from build123d import *

# Parameters (mm, degrees)
SKETCH1_R           = 2.5
BOSS_EXTRUDE1_DEPTH = 10


with BuildPart() as part:
    # Sketch1 → Boss-Extrude1 (new body)
    with BuildSketch(Plane.XY):
        with BuildLine():
            Line((-30, 0), (-22.5, 0))
            Line((-22.5, 0), (-22.5, 1))
            ThreePointArc((-22.5, 1), (-22.207106781, 1.707106781), (-21.5, 2))
            Line((-21.5, 2), (-9, 2))
            Line((-9, 2), (-9, 3))
            ThreePointArc((-9, 3), (-8.707106781, 3.707106781), (-8, 4))
            Line((-8, 4), (8, 4))
            ThreePointArc((8, 4), (8.707106781, 3.707106781), (9, 3))
            Line((9, 3), (9, 2))
            Line((9, 2), (21.5, 2))
            ThreePointArc((21.5, 2), (22.207106781, 1.707106781), (22.5, 1))
            Line((22.5, 1), (22.5, 0))
            Line((22.5, 0), (30, 0))
            Line((30, 0), (24.933748499, 30.8112495))
            ThreePointArc((24.933748499, 30.8112495), (23.236027851, 33.811577593), (20, 35))
            Line((20, 35), (16, 35))
            Line((16, 35), (16, 29))
            ThreePointArc((16, 29), (15.414213562, 27.585786438), (14, 27))
            Line((14, 27), (10, 27))
            ThreePointArc((10, 27), (0, 17), (-10, 27))
            Line((-10, 27), (-14, 27))
            ThreePointArc((-14, 27), (-15.414213562, 27.585786438), (-16, 29))
            Line((-16, 29), (-16, 35))
            Line((-16, 35), (-20, 35))
            ThreePointArc((-20, 35), (-23.236027851, 33.811577593), (-24.933748499, 30.8112495))
            Line((-24.933748499, 30.8112495), (-30, 0))
        make_face()
        with Locations((-20, 30)):
            Circle(SKETCH1_R, mode=Mode.SUBTRACT)
        with Locations(Location((20, 30, 0), (0, 0, 180))):
            Circle(SKETCH1_R, mode=Mode.SUBTRACT)
    extrude(amount=BOSS_EXTRUDE1_DEPTH)


solid = part.part
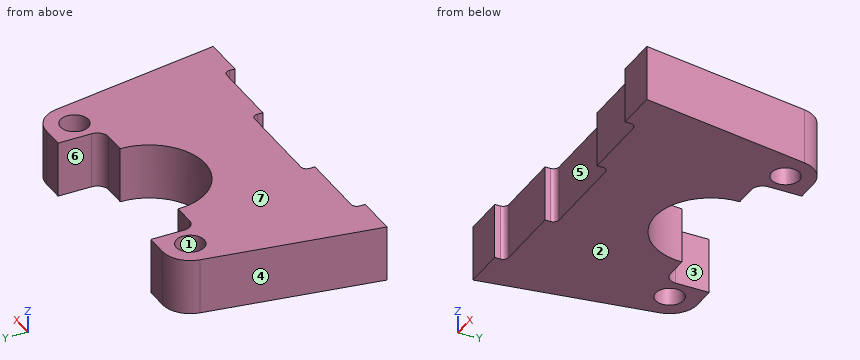
Geometry: final body of the model. Coordinates: model frame, mm. Face numbers are marked on the shaded views. A direction names the side the tool comes from. Round coordinates to 2 decimals unless told otherwise and drop trailing zeros. Order: outer loops, then holes, each group sorted by start corner. A loop starts at its lowest first (then second) coordinate and runs counter-clockwise, first axis right, second up. Notation, with made-up numbers: (46, -20.5) -> (51, -20.5) arc R14 cw to (51, 3.5) -> close; hole circle Ø3 at (54, -16.5). An arc over 180 degrees is marked (long way). Put each result on its own line as item: value. Start each with the question number.
Q1. Pull-direction query (X, two-part tool) for the marked faces 1, 2, 3 and 4; classes: +X half, -X half, draft (parallel to the pull), parting line (faces both ways), or undercut.
Q2. Reachability of the marked faces 5, 6 and 7 from +Z, -Z, +X, -X, +Y, -Y: full face, straight path, thin tool, end or side. Return the list, or none.
Q3. Section B-B on y = 25.5. Return the cut outline in (x, z), and give its area (3 significant figures).
Q4. Line query: probe 1 along Y at (x, z) = (-20, 4.75); probe 2 along X at (y, z) = (31, 2.5); probe 3 along X at (y, z) = (28, 1.5). Output: solid intervals per line, ascending.
Q5. Section D-D on x = 12. Return the cut outline in (y, z), and give its area (3 significant figures).
Q6. Section C-C on y = 30. Return the cut outline in (x, z), and give its area (3 significant figures).
Q7. First-contact query: pin 1 (5 mm diameter, centred on y = 33, z = 4.5, fed in from -X); pin 2 (4.5 mm diameter, centred on x = 12.5, z = 2.5, fed in from +Y); pin 3 (0.8 mm diameter, centred on y = 0.5, z = 4, fed in from +X); pin 4 (3 mm diameter, centred on x = -20, y = 30, fed in from +Z). Flat tips, straight axial feed; report the tip coordinate or a pass-through.
Q8. Section A-A on z = 1.25. Return the cut outline in (x, y).
Ans:
1. face 1: undercut
1. face 2: draft
1. face 3: undercut
1. face 4: -X half
2. face 5: +Z, -Z, -Y
2. face 6: +Z, -Z, +Y
2. face 7: +Z, +X, -X, +Y, -Y
3. outline: (-25.81, 0) -> (-9.89, 0) -> (-9.89, 10) -> (-25.81, 10) -> close; (9.89, 0) -> (25.81, 0) -> (25.81, 10) -> (9.89, 10) -> close
3. area: 318 mm2
4. probe 1: y = 2 to 27.5, 32.5 to 35
4. probe 2: x = -24.9 to -22.29, -17.71 to -16, 16 to 17.71, 22.29 to 24.9
4. probe 3: x = -25.4 to -21.5, -18.5 to -15.73, 15.73 to 18.5, 21.5 to 25.4
5. outline: (2, 0) -> (27, 0) -> (27, 10) -> (2, 10) -> close
5. area: 250 mm2
6. outline: (-25.07, 0) -> (-22.5, 0) -> (-22.5, 10) -> (-25.07, 10) -> close; (-17.5, 0) -> (-16, 0) -> (-16, 10) -> (-17.5, 10) -> close; (16, 0) -> (17.5, 0) -> (17.5, 10) -> (16, 10) -> close; (22.5, 0) -> (25.07, 0) -> (25.07, 10) -> (22.5, 10) -> close
6. area: 81.3 mm2
7. pin 1: stops at x = -24.98
7. pin 2: stops at y = 27.15
7. pin 3: stops at x = 29.98
7. pin 4: passes through
8. outline: (-30, 0) -> (-22.5, 0) -> (-22.5, 1) arc R1 cw to (-21.5, 2) -> (-9, 2) -> (-9, 3) arc R1 cw to (-8, 4) -> (8, 4) arc R1 cw to (9, 3) -> (9, 2) -> (21.5, 2) arc R1 cw to (22.5, 1) -> (22.5, 0) -> (30, 0) -> (24.93, 30.81) arc R5 ccw to (20, 35) -> (16, 35) -> (16, 29) arc R2 cw to (14, 27) -> (10, 27) arc R10 cw to (-10, 27) -> (-14, 27) arc R2 cw to (-16, 29) -> (-16, 35) -> (-20, 35) arc R5 ccw to (-24.93, 30.81) -> close; hole circle Ø5 at (-20, 30); hole circle Ø5 at (20, 30)
